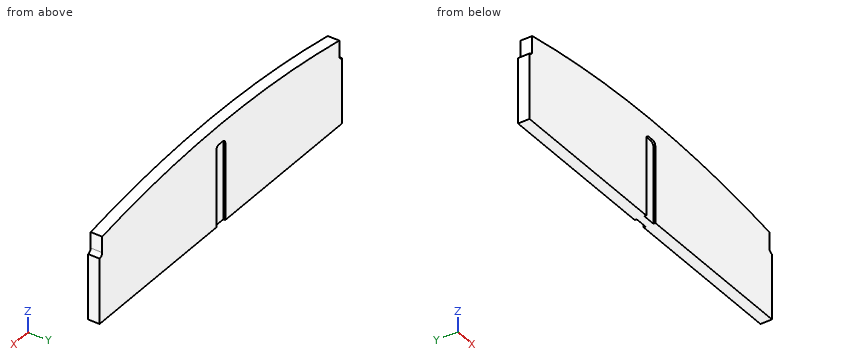
from build123d import *

# Parameters (mm, degrees)
F1_DEPTH = 9.50849
F3_DEPTH = 3.175
F5_DEPTH = 3.175


with BuildPart() as f1:
    # F0 (on Front) → F1 (new body, symmetric)
    with BuildSketch(Plane.XZ):
        with BuildLine():
            Line((-292.100635, -70.246875), (285.750635, -70.246875))
            Line((285.750635, -70.246875), (285.750635, 37.703125))
            ThreePointArc((285.750635, 37.703125), (281.2605069395, 39.5629969395), (279.400635, 44.053125))
            Line((279.400635, 44.053125), (279.400635, 70.246875))
            ThreePointArc((279.400635, 70.246875), (-3.175, 94.3266404561), (-285.750635, 70.246875))
            Line((-285.750635, 70.246875), (-285.750635, 44.053125))
            ThreePointArc((-285.750635, 44.053125), (-287.6105069395, 39.5629969395), (-292.100635, 37.703125))
            Line((-292.100635, 37.703125), (-292.100635, -70.246875))
        make_face()
    extrude(amount=F1_DEPTH, both=True)

    # F2 (on face) → F3 (cut)
    with BuildSketch(Plane.XZ.offset(9.50849)):
        with BuildLine():
            Line((1.190625, 63.103125), (-7.540625, 63.103125))
            ThreePointArc((-7.540625, 63.103125), (-12.0307530605, 61.2432530605), (-13.890625, 56.753125))
            Line((-13.890625, 56.753125), (-13.890625, -70.246875))
            Line((-13.890625, -70.246875), (7.540625, -70.246875))
            Line((7.540625, -70.246875), (7.540625, 56.753125))
            ThreePointArc((7.540625, 56.753125), (5.6807530605, 61.2432530605), (1.190625, 63.103125))
        make_face()
    extrude(amount=-F3_DEPTH, mode=Mode.SUBTRACT)

    # F4 (on face) → F5 (cut)
    with BuildSketch(Plane(origin=(0, 9.50849, 0), x_dir=(-1, 0, 0), z_dir=(0, 1, 0))):
        with BuildLine():
            Line((-7.540625, 56.753125), (-7.540625, -70.246875))
            Line((-7.540625, -70.246875), (13.890625, -70.246875))
            Line((13.890625, -70.246875), (13.890625, 56.753125))
            ThreePointArc((13.890625, 56.753125), (12.0307530605, 61.2432530605), (7.540625, 63.103125))
            Line((7.540625, 63.103125), (-1.190625, 63.103125))
            ThreePointArc((-1.190625, 63.103125), (-5.6807530605, 61.2432530605), (-7.540625, 56.753125))
        make_face()
    extrude(amount=-F5_DEPTH, mode=Mode.SUBTRACT)


solid = f1.part
Design review of the part built by this model. Coordinates are the model's own, in mm. Give positions to 0.01 mm unless a question says otherwise; leave off trailing zeros. Order: outer loops, then holes, each group sorted by start corner. A loop starts at its lowest first (then second) coordinate and runs counter-clockwise, first axis right, second up. Notation, with made-up numbers: (75, -24.5) - (114, -24.5) arc R19 ccw to (114, -19.5) - close; hole circle Ø5 at (-6, 2.25). An arc over 180 degrees is marked (long way). Write item = value, one per line. Start each with the question number.
Q1. We need section A-A on y = -3. State the section outline as (x, z) points (3 decimals), plus the area to 3 significant figures.
Q2. To check wall thickness, follow L1, parallel to X at y = -6.75, z = 49; L2, parallel to Z at x = -6.5, y = -3.75; L3, parallel to X at y = 7, z = 68. State the ranges of each line that lie inside material, in increasing order. Write a range as from..to.
Q3. Clearance check with flat-ended pins moving along their axes: pin 1 Ø6.5 at (x, z) = (-3.5, -32.5) entering from -Y; pin 2 Ø1 at (x, y) = (-3.5, -8) entering from -Z; pin 3 Ø6.5 at (x, z) = (-2, 0.5) entering from +Y. State where each tip first meets the part, or that it passes through.
Q4. We need section C-C on x = 225.5. State the section outline as (y, z) points.
Q5. We need section B-B on x = 107.5. State the section outline as (y, z) points, plus the area to 3 significant figures.
Working result:
q1.outline = (-292.101, -70.247) - (285.751, -70.247) - (285.751, 37.703) arc R6.35 cw to (279.401, 44.053) - (279.401, 70.247) arc R1670.05 ccw to (-285.751, 70.247) - (-285.751, 44.053) arc R6.35 cw to (-292.101, 37.703) - close
q1.area = 89,900 mm²
q2.L1 = -285.75..-13.89, 7.54..279.4
q2.L2 = -70.25..94.32
q2.L3 = -285.75..279.4
q3.pin_1 = -6.33
q3.pin_2 = 63.1
q3.pin_3 = 6.33
q4.outline = (-9.51, -70.25) - (9.51, -70.25) - (9.51, 78.6) - (-9.51, 78.6) - close
q5.outline = (-9.51, -70.25) - (9.51, -70.25) - (9.51, 90.66) - (-9.51, 90.66) - close
q5.area = 3,060 mm²
